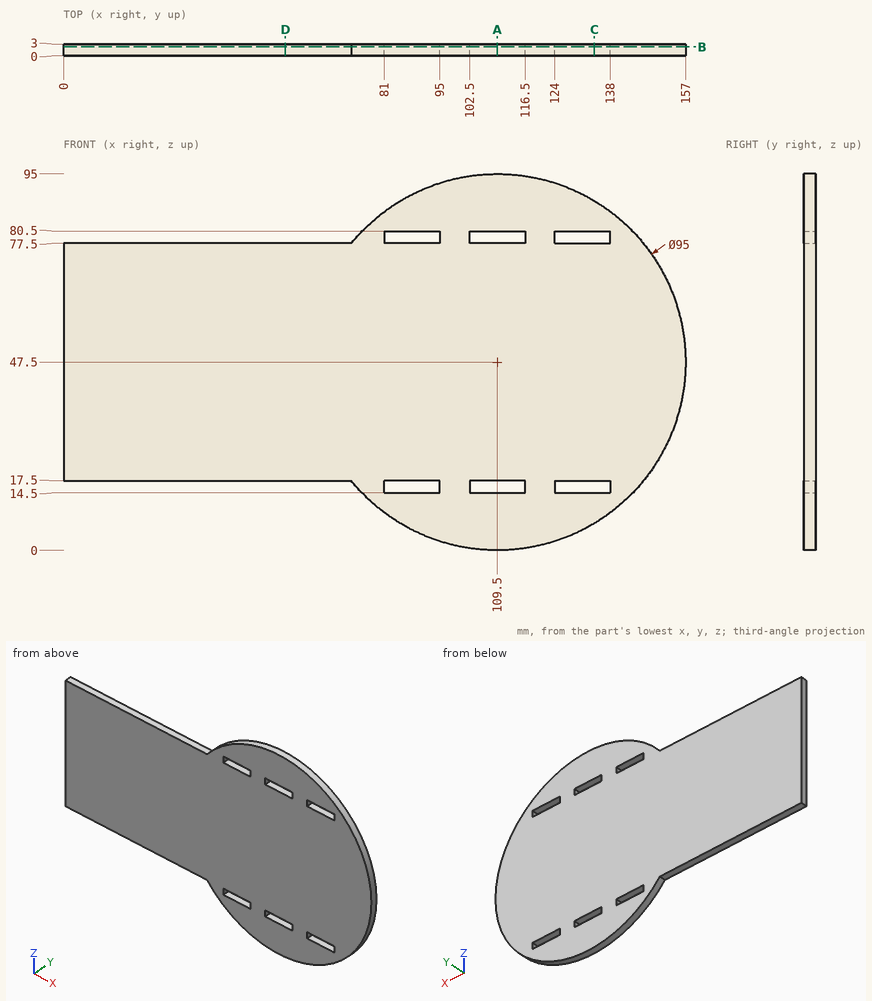
Drawing for the job (mm, zero at the part's lowest x, y, z). Give positions to 0.01 mm unless a question says otherwise; leave off trailing zeros. Write each loop counter-clockwise with the first axis right and the second up, starting at its lowest first coordinate (ties: lowest second). Pieces come first, ordered by that corner, then holes. Notation, with made-up numbers: (-34, -15.5) -> (7, -15.5) arc R24 cw to (7, 13.5) -> close; hole circle Ø9 at (70, -9.5). An arc over 180 degrees is marked (long way). Put each result on its own line as item: value. Start each with the question number.
Item 1: Cut at B-B (y = 2.3). List the corners of the cut face in (x, z), then the cut area to 3 significant figures.
Item 2: Cut at C-C (x = 134). List the corners of the cut face in (y, z), then the cut area to 3 significant figures.
Item 3: Cut at D-D (x = 56). List the corners of the cut face in (y, z), then the cut area to 3 significant figures.
Item 4: Pin check, flat tips, straight feed: pin 1 Ø1.5 at (x, y) = (130.5, 2) entering from +Z; pin 2 Ø1.5 at (y, z) = (1.5, 16.5) entering from +X; pin 3 Ø1.5 at (y, z) = (1, 79) entering from +X. Stop position of each tip, or through.
Item 5: Wall check: L1, parallel to Z at x = 83, y = 0.9; L2, parallel to X at y = 0.4, z = 16; L3, parallel to Z at x = 127, y = 0.85. Give the ranges that are in metal, low to high. Write a range as [from, to].
Item 6: Cut at A-A (x = 109.5). List the corners of the cut face in (y, z), then the cut area to 3 significant figures.
Answer list:
1. outline: (0, 17.5) -> (72.67, 17.5) arc R47.5 ccw (long way) to (72.67, 77.5) -> (0, 77.5) -> close; hole (81, 14.5) -> (95, 14.5) -> (95, 17.5) -> (81, 17.5) -> close; hole (81, 77.5) -> (95, 77.5) -> (95, 80.5) -> (81, 80.5) -> close; hole (102.5, 14.5) -> (116.5, 14.5) -> (116.5, 17.5) -> (102.5, 17.5) -> close; hole (102.5, 77.5) -> (116.5, 77.5) -> (116.5, 80.5) -> (102.5, 80.5) -> close; hole (124, 14.5) -> (138, 14.5) -> (138, 17.5) -> (124, 17.5) -> close; hole (124, 77.5) -> (138, 77.5) -> (138, 80.5) -> (124, 80.5) -> close
1. area: 10,800 mm2
2. outline: (0, 6.81) -> (3, 6.81) -> (3, 14.5) -> (0, 14.5) -> close; (0, 17.5) -> (3, 17.5) -> (3, 77.5) -> (0, 77.5) -> close; (0, 80.5) -> (3, 80.5) -> (3, 88.19) -> (0, 88.19) -> close
2. area: 226 mm2
3. outline: (0, 17.5) -> (3, 17.5) -> (3, 77.5) -> (0, 77.5) -> close
3. area: 180 mm2
4. pin 1: stops at z = 90.47
4. pin 2: stops at x = 146.12
4. pin 3: stops at x = 145.7
5. L1: z = [8.08, 14.5], [17.5, 77.5], [80.5, 86.92]
5. L2: x = [73.95, 81], [95, 102.5], [116.5, 124], [138, 145.05]
5. L3: z = [3.34, 14.5], [17.5, 77.5], [80.5, 91.66]
6. outline: (0, 0) -> (3, 0) -> (3, 14.5) -> (0, 14.5) -> close; (0, 17.5) -> (3, 17.5) -> (3, 77.5) -> (0, 77.5) -> close; (0, 80.5) -> (3, 80.5) -> (3, 95) -> (0, 95) -> close
6. area: 267 mm2
